from build123d import *

# Parameters (mm, degrees)
F1_DEPTH      = 16
F2_W          = 2.8
F2_H          = 5
F3_DEPTH      = 33.601
F4_W          = 5
F4_H          = 26
F5_DEPTH      = 10.001
F7_DEPTH      = 16
F8_R          = 1.5
F9_SIZE       = 2
F10_T1_DEPTH  = 5.5
F10_T3_DEPTH  = 5.5
F10_T8_DEPTH  = 11.5355339059
F10_T13_DEPTH = 11.5355339059
F10_T15_DEPTH = 21
F10_T17_DEPTH = 18.0710678119
F10_T19_DEPTH = 6.3867513459
F10_T21_DEPTH = 6.3867513459


# Not quite as in the source:
# - a fillet or chamfer that OpenCascade refuses, or shapes differently, is made with other operations: its cross-section is extruded or revolved along the edge and cut away or added


with BuildPart() as f1:
    # F0 (on Front) → F1 (new body)
    with BuildSketch(Plane.XZ):
        Polygon((-3.6, 30.8), (-6.4, 30.8), (-6.4, 27.829016319), (-1.5, 25), (-1.5, 5), (-6.4, 2.170983681), (-6.4, -2.8), (-3.6, -2.8), (-3.6, 0), (3.6, 0), (3.6, -2.8), (6.4, -2.8), (6.4, 2.170983681), (1.5, 5), (1.5, 25), (6.4, 27.829016319), (6.4, 30.8), (3.6, 30.8), (3.6, 30), (-3.6, 30), align=None)
    extrude(amount=F1_DEPTH)

    # F2 (on face) → F3 (cut, through all)
    with BuildSketch(Plane.XY.offset(30.8)):
        with Locations((-5, -8)):
            Rectangle(F2_W, F2_H)
        with Locations((5, -8)):
            Rectangle(F2_W, F2_H)
    extrude(amount=-F3_DEPTH, mode=Mode.SUBTRACT)

    # F4 (on face) → F5 (cut, through all)
    with BuildSketch(Plane(origin=(-3.6, 0, 0), x_dir=(0, -1, 0), z_dir=(-1, 0, 0))):
        with Locations((8, 15)):
            Rectangle(F4_W, F4_H)
    extrude(amount=-F5_DEPTH, mode=Mode.SUBTRACT)

    # F6 (on face) → F7 (join, through all)
    with BuildSketch(Plane.XZ.offset(16)):
        Polygon((-8.4142135624, 6), (-4.5857864376, 6), (1.5, 12.0857864376), (1.5, 23.6), (-11.5, 23.6), (-11.5, 9.0857864376), align=None)
        Polygon((-10.5, 9.5), (-10.5, 22.6), (-2.5, 22.6), (-2.5, 9.5), (-5, 7), (-8, 7), align=None, mode=Mode.SUBTRACT)
    extrude(amount=-F7_DEPTH)

    # F8
    f8_edges = [f1.edges().sort_by_distance(p)[0] for p in [
        (3.6, -8, 2),
        (3.6, -8, 28),
        (-3.6, -8, 28),
        (-3.6, -8, 2),
    ]]
    fillet(f8_edges, radius=F8_R)

    # F9
    f9_edges = [f1.edges().sort_by_distance(p)[0] for p in [
        (6.4, -10.5, -0.314508),
        (6.4, -5.5, -0.314508),
        (6.4, -10.5, 29.314508),
        (6.4, -5.5, 29.314508),
        (-6.4, -5.5, -0.314508),
        (-6.4, -10.5, -0.314508),
        (-6.4, -5.5, 29.314508),
        (-6.4, -10.5, 29.314508),
    ]]
    chamfer(f9_edges, length=F9_SIZE)

    # F10: fillet of radius 1 on 24 edges, made by hand

    # F10_s2 → F10_t1 (join)
    with BuildSketch(Plane.XZ.offset(10.5)):
        with BuildLine():
            ThreePointArc((-3.2071067812, 7.3786796564), (-2.1173165676, 7.5954524078), (-1.5, 6.6715728753))
            Line((-1.5, 6.6715728753), (-1.5, 9.0857864376))
            Line((-1.5, 9.0857864376), (-3.2071067812, 7.3786796564))
        make_face()
        with BuildLine():
            ThreePointArc((-1.5, 24.6), (-1.7928932188, 23.8928932188), (-2.5, 23.6))
            Line((-2.5, 23.6), (-1.5, 23.6))
            Line((-1.5, 23.6), (-1.5, 24.6))
        make_face()
        with BuildLine():
            ThreePointArc((1.5, 5.5773502692), (1.6339745962, 5.0773502692), (2, 4.7113248654))
            Line((2, 4.7113248654), (1.5, 5))
            Line((1.5, 5), (1.5, 5.5773502692))
        make_face()
        with BuildLine():
            ThreePointArc((1.5, 24.4226497308), (1.6339745962, 24.9226497308), (2, 25.2886751346))
            Line((2, 25.2886751346), (1.5, 25))
            Line((1.5, 25), (1.5, 24.4226497308))
        make_face()
        with BuildLine():
            ThreePointArc((-1.5, 5.5773502692), (-1.6339745962, 5.0773502692), (-2, 4.7113248654))
            Line((-2, 4.7113248654), (-1.5, 5))
            Line((-1.5, 5), (-1.5, 5.5773502692))
        make_face()
        with BuildLine():
            ThreePointArc((-2, 25.2886751346), (-1.6339745962, 24.9226497308), (-1.5, 24.4226497308))
            Line((-1.5, 24.4226497308), (-1.5, 25))
            Line((-1.5, 25), (-2, 25.2886751346))
        make_face()
    extrude(amount=F10_T1_DEPTH)

    # F10_s4 → F10_t3 (join)
    with BuildSketch(Plane.XZ):
        with BuildLine():
            ThreePointArc((-3.2071067812, 7.3786796564), (-2.1173165676, 7.5954524078), (-1.5, 6.6715728753))
            Line((-1.5, 6.6715728753), (-1.5, 9.0857864376))
            Line((-1.5, 9.0857864376), (-3.2071067812, 7.3786796564))
        make_face()
        with BuildLine():
            ThreePointArc((-2.5, 23.6), (-1.7928932188, 23.8928932188), (-1.5, 24.6))
            Line((-1.5, 24.6), (-1.5, 23.6))
            Line((-1.5, 23.6), (-2.5, 23.6))
        make_face()
        with BuildLine():
            ThreePointArc((1.5, 5.5773502692), (1.6339745962, 5.0773502692), (2, 4.7113248654))
            Line((2, 4.7113248654), (1.5, 5))
            Line((1.5, 5), (1.5, 5.5773502692))
        make_face()
        with BuildLine():
            ThreePointArc((1.5, 24.4226497308), (1.6339745962, 24.9226497308), (2, 25.2886751346))
            Line((2, 25.2886751346), (1.5, 25))
            Line((1.5, 25), (1.5, 24.4226497308))
        make_face()
        with BuildLine():
            ThreePointArc((-1.5, 5.5773502692), (-1.6339745962, 5.0773502692), (-2, 4.7113248654))
            Line((-2, 4.7113248654), (-1.5, 5))
            Line((-1.5, 5), (-1.5, 5.5773502692))
        make_face()
        with BuildLine():
            ThreePointArc((-1.5, 24.4226497308), (-1.6339745962, 24.9226497308), (-2, 25.2886751346))
            Line((-2, 25.2886751346), (-1.5, 25))
            Line((-1.5, 25), (-1.5, 24.4226497308))
        make_face()
    extrude(amount=F10_T3_DEPTH)


with BuildPart() as f10_tool6:
    # F10_s7 → F10_t8 (new body)
    with BuildSketch(Plane.XZ.offset(16)):
        with BuildLine():
            ThreePointArc((-3.2071067812, 7.3786796564), (-2.1173165676, 7.5954524078), (-1.5, 6.6715728753))
            Line((-1.5, 6.6715728753), (-1.5, 9.0857864376))
            Line((-1.5, 9.0857864376), (-3.2071067812, 7.3786796564))
        make_face()
    extrude(amount=-F10_T8_DEPTH)

    split(bisect_by=Plane.XZ.offset(5.5), keep=Keep.BOTTOM)


with BuildPart() as f1_1:
    add(f1.part)

    # F10_t5: union F10_tool6
    add(f10_tool6.part)


with BuildPart() as f10_tool11:
    # F10_s12 → F10_t13 (new body)
    with BuildSketch(Plane.XZ.offset(11.5355339059)):
        with BuildLine():
            ThreePointArc((-3.2071067812, 7.3786796564), (-2.1173165676, 7.5954524078), (-1.5, 6.6715728753))
            Line((-1.5, 6.6715728753), (-1.5, 9.0857864376))
            Line((-1.5, 9.0857864376), (-3.2071067812, 7.3786796564))
        make_face()
    extrude(amount=-F10_T13_DEPTH)

    split(bisect_by=Plane.XZ.offset(10.5), keep=Keep.TOP)


with BuildPart() as f1_2:
    add(f1_1.part)

    # F10_t10: union F10_tool11
    add(f10_tool11.part)

    # F10_s16 → F10_t15 (cut)
    with BuildSketch(Plane.XZ.offset(-2.5)):
        with BuildLine():
            ThreePointArc((-11.5, 22.6), (-11.2071067812, 23.3071067812), (-10.5, 23.6))
            Line((-10.5, 23.6), (-11.5, 23.6))
            Line((-11.5, 23.6), (-11.5, 22.6))
        make_face()
    extrude(amount=F10_T15_DEPTH, mode=Mode.SUBTRACT)

    # F10_s18 → F10_t17 (cut)
    with BuildSketch(Plane.XZ.offset(-1.0355339059)):
        with BuildLine():
            ThreePointArc((-11.2071067812, 8.7928932188), (-11.4238795325, 9.1173165676), (-11.5, 9.5))
            Line((-11.5, 9.5), (-11.5, 9.0857864376))
            Line((-11.5, 9.0857864376), (-11.2071067812, 8.7928932188))
        make_face()
        with BuildLine():
            ThreePointArc((-8, 6), (-8.3826834324, 6.0761204675), (-8.7071067812, 6.2928932188))
            Line((-8.7071067812, 6.2928932188), (-8.4142135624, 6))
            Line((-8.4142135624, 6), (-8, 6))
        make_face()
        with BuildLine():
            ThreePointArc((-4.2928932188, 6.2928932188), (-4.6173165676, 6.0761204675), (-5, 6))
            Line((-5, 6), (-4.5857864376, 6))
            Line((-4.5857864376, 6), (-4.2928932188, 6.2928932188))
        make_face()
    extrude(amount=F10_T17_DEPTH, mode=Mode.SUBTRACT)

    # F10_s20 → F10_t19 (cut)
    with BuildSketch(Plane.XZ.offset(11.056624327)):
        with BuildLine():
            ThreePointArc((-6.4, 1.5936334118), (-6.2660254038, 2.0936334118), (-5.9, 2.4596588156))
            Line((-5.9, 2.4596588156), (-6.4, 2.170983681))
            Line((-6.4, 2.170983681), (-6.4, 1.5936334118))
        make_face()
        with BuildLine():
            ThreePointArc((-6.4, 28.4063665882), (-6.2660254038, 27.9063665882), (-5.9, 27.5403411844))
            Line((-5.9, 27.5403411844), (-6.4, 27.829016319))
            Line((-6.4, 27.829016319), (-6.4, 28.4063665882))
        make_face()
        with BuildLine():
            ThreePointArc((6.4, 28.4063665882), (6.2660254038, 27.9063665882), (5.9, 27.5403411844))
            Line((5.9, 27.5403411844), (6.4, 27.829016319))
            Line((6.4, 27.829016319), (6.4, 28.4063665882))
        make_face()
        with BuildLine():
            ThreePointArc((5.9, 2.4596588156), (6.2660254038, 2.0936334118), (6.4, 1.5936334118))
            Line((6.4, 1.5936334118), (6.4, 2.170983681))
            Line((6.4, 2.170983681), (5.9, 2.4596588156))
        make_face()
    extrude(amount=F10_T19_DEPTH, mode=Mode.SUBTRACT)

    # F10_s22 → F10_t21 (cut)
    with BuildSketch(Plane.XZ.offset(-1.443375673)):
        with BuildLine():
            ThreePointArc((-6.4, 1.5936334118), (-6.2660254038, 2.0936334118), (-5.9, 2.4596588156))
            Line((-5.9, 2.4596588156), (-6.4, 2.170983681))
            Line((-6.4, 2.170983681), (-6.4, 1.5936334118))
        make_face()
        with BuildLine():
            ThreePointArc((-5.9, 27.5403411844), (-6.2660254038, 27.9063665882), (-6.4, 28.4063665882))
            Line((-6.4, 28.4063665882), (-6.4, 27.829016319))
            Line((-6.4, 27.829016319), (-5.9, 27.5403411844))
        make_face()
        with BuildLine():
            ThreePointArc((6.4, 28.4063665882), (6.2660254038, 27.9063665882), (5.9, 27.5403411844))
            Line((5.9, 27.5403411844), (6.4, 27.829016319))
            Line((6.4, 27.829016319), (6.4, 28.4063665882))
        make_face()
        with BuildLine():
            ThreePointArc((5.9, 2.4596588156), (6.2660254038, 2.0936334118), (6.4, 1.5936334118))
            Line((6.4, 1.5936334118), (6.4, 2.170983681))
            Line((6.4, 2.170983681), (5.9, 2.4596588156))
        make_face()
    extrude(amount=F10_T21_DEPTH, mode=Mode.SUBTRACT)


solid = f1_2.part
Source: CAD feature listing. Evaluate the final solid. Frame: model axes, mm. A direction names the side the tool comes from. Round coordinates to 2 decimals unless told otherwise and drop trailing zeros. Loops run counter-clockwise (first coordinate to the right, second up) from the corner with the lowest first, then second, coordinate; pieces in that order, holes last. Notation, with made-up numbers: M 7,29.25 L 44,29.25 A5 ccw 44,37.25 Z; hole C -36,34 d11. An arc over 180 degrees is marked long. Return JSON: item names as keys, results as strings. Group by question number.
1. Mould query, pull axis X, two halves, no side actions, for faces 1 (the face through (-3.98, -2.71, 26.43)), 2 (the face through (0, -5.5, 27)), 3 (the face through (3.6, -13, -1)), 4 (the face through (3.6, -2.7, 30.4)). Classes: released by +X, released by -X, zero draft, split by the parting line, or undercut.
2. Section query B-B on z = 20. Output: boundary loops of the cut face in (x, y).
3. Section query D-D on x = -0.75. Output: boundary loops of the cut face in (y, z).
4. Reachability of faces 5 (the face through (-3.15, -8.04, 28.43)), 6 (the face through (-6.4, -14, 30)), 7 (the face through (6.27, -13.97, 27.91)) from +Z, -Z, +X, -X, +Y, -Y: full face, straight path, thin tool, end or side. Return the list, or none.
5. Section query A-A on y = -7.25. Output: boundary loops of the cut face in (x, z).
6. Pin query (flat end, axial travel): pin 1 (8 mm diameter, centred on y = -9, z = 16, fed in from +X); pin 2 (2 mm diameter, centred on x = -5, z = 9, fed in from +Y); pin 3 (3.5 mm diameter, centred on x = -0.5, y = -4.5, fed in from +Z); pin 4 (1.4 mm diameter, centred on y = -2, z = -1.5, fed in from -X). Return the tip coordinate at first contact, or that it passes through.
7. Material intervals for line 1 along Z through (x, y) = (-1.25, -10); line 2 along X through (y, z) = (-14.75, 13); line 3 along Z through (x, y) = (-3, -6.75), sorted ascending. Write a range as from..to.
8. Section query C-C on x = -10. Output: boundary loops of the cut face in (y, z).
Checks:
{
 "1": {"face 1": "released by -X", "face 2": "zero draft", "face 3": "undercut", "face 4": "undercut"},
 "2": {"outline": "M -11.5,-16 L -10.5,-16 L -10.5,0 L -11.5,0 Z; M -2.5,-16 L 1.5,-16 L 1.5,0 L -2.5,0 Z"},
 "3": {"outline": "M -16,0 L 0,0 L 0,30 L -16,30 Z; hole M -10.5,2 L -5.5,2 L -5.5,9.84 L -10.5,9.84 Z; hole M -10.5,23.6 L -5.5,23.6 L -5.5,28 L -10.5,28 Z"},
 "4": {"face 5": "-X", "face 6": "+Z, -X, +Y, -Y", "face 7": "+X, +Y, -Y"},
 "5": {"outline": "M -11.5,9.5 A1 ccw -11.21,8.79 L -8.71,6.29 A1 ccw -8,6 L -5,6 A1 ccw -4.29,6.29 L 1.5,12.09 L 1.5,23.6 L -10.5,23.6 A1 ccw -11.5,22.6 Z; M -3.6,0 L 3.6,0 L 3.6,0.5 A1.5 ccw 2.1,2 L -2.1,2 A1.5 ccw -3.6,0.5 Z; M -3.6,29.5 A1.5 ccw -2.1,28 L 2.1,28 A1.5 ccw 3.6,29.5 L 3.6,30 L -3.6,30 Z; hole M -10.5,9.5 L -8,7 L -5,7 L -2.5,9.5 L -2.5,22.6 L -10.5,22.6 Z"},
 "6": {"pin 1": "stops at x = 1.5", "pin 2": "passes through", "pin 3": "stops at z = 30", "pin 4": "stops at x = -6.4"},
 "7": {"line 1": "z = 0..2, 9.34..23.6, 28..30", "line 2": "x = -11.5..-10.5, -2.5..1.5", "line 3": "z = 0..1.7, 7.59..9, 22.6..23.6, 28.3..30"},
 "8": {"outline": "M -16,7.59 L 0,7.59 L 0,9 L -16,9 Z; M -16,22.6 L 0,22.6 L 0,23.6 L -16,23.6 Z"}
}
